Autodesk Inventor part; units mm, degrees
ref_plane "YZ Plane" through (0, 0, 0) normal (1, 0, 0) x (0, 1, 0)
ref_plane "XZ Plane" through (0, 0, 0) normal (0, 1, 0) x (-1, 0, 0)
ref_plane "XY Plane" through (0, 0, 0) normal (0, 0, 1) x (1, 0, 0)
sketch "スケッチ1" plane through (0, 0, 0) normal (0, 0, 1) x (1, 0, 0)
  line L0 (-28, -35) -> (28, -35) construction
  line L1 (28, -35) -> (28, 35) construction
  line L2 (28, 35) -> (-28, 35) construction
  line L3 (-28, 35) -> (-28, -35) construction
  line L4 (-28, -35) -> (28, 35) construction
  line L5 (28, -35) -> (-28, 35) construction
  line L6 (-28, 22.1) -> (-28, 35)
  line L7 (-28, 35) -> (28, 35)
  line L8 (28, 35) -> (28, 22.1)
  line L9 (-28, 20) -> (-33, 20)
  line L10 (-33, 20) -> (-33, -20)
  line L11 (-33, -20) -> (-28, -20)
  line L12 (-28, -22.1) -> (-28, -35)
  line L13 (-28, -35) -> (28, -35)
  line L14 (28, -35) -> (28, -22.1)
  line L15 (28, 20) -> (33, 20)
  line L16 (33, 20) -> (33, -20)
  line L17 (33, -20) -> (28, -20)
  arc A0 (-28, 20) -> (-28, 22.1) centre (-28, 21.05) ccw
  arc A1 (-28, -22.1) -> (-28, -20) centre (-28, -21.05) ccw
  arc A2 (28, -20) -> (28, -22.1) centre (28, -21.05) ccw
  line L18 (0, 0) -> (0, 35) construction
  line L19 (0, 0) -> (28, 0) construction
  arc A3 (28, 22.1) -> (28, 20) centre (28, 21.05) ccw
  dimension "d9" = 56
  dimension "d12" = 70
  dimension "d13" = 15
  dimension "d39" = 15
  dimension "d40" = 1.05
  dimension "d41" = 5
extrude "押し出し1" add sketch "スケッチ1" along normal blind 5
sketch "スケッチ2" plane through (0, 0, 5) normal (0, 0, 1) x (1, 0, 0)
  line L0 (-28, 35) -> (-28, 22.1)
  line L1 (28, 35) -> (-28, 35)
  line L2 (-67.7785, 43.014) -> (-28, 43.014)
  line L3 (-28, 43.014) -> (-28, -43.014)
  line L4 (-28, -43.014) -> (-67.7785, -43.014)
  line L5 (-67.7785, -43.014) -> (-67.7785, 43.014)
  line L6 (67.7785, 43.014) -> (28, 43.014)
  line L7 (28, 43.014) -> (28, -43.014)
  line L8 (28, -43.014) -> (67.7785, -43.014)
  line L9 (67.7785, -43.014) -> (67.7785, 43.014)
  line L10 (0, 0) -> (0, 35) construction
  line L11 (0, 0) -> (33, 0) construction
  line L12 (33, 20) -> (33, -20) construction
extrude "押し出し2" cut sketch "スケッチ2" against normal blind 2.5
sketch "スケッチ3" plane through (0, 0, 5) normal (0, 0, 1) x (1, 0, 0)
  line L0 (28, 35) -> (-28, 35)
  line L1 (-28, 35) -> (-28, 22.1)
  line L2 (-20, -27) -> (20, -27)
  line L3 (20, -27) -> (20, 27)
  line L4 (20, 27) -> (-20, 27)
  line L5 (-20, 27) -> (-20, -27)
  line L6 (-20, -27) -> (20, 27) construction
  line L7 (20, -27) -> (-20, 27) construction
  point P0 (0, 0)
  dimension "d47" = 8
  dimension "d48" = 8
extrude "押し出し3" cut sketch "スケッチ3" against normal blind 10
fillet "フィレット1" radius 10 4 edges at (-20, 27, 2.5) (20, 27, 2.5) (20, -27, 2.5) (-20, -27, 2.5)
equation "\"d12\" = d18"
equation "\"d13\" = d28"
equation "\"d39\" = d13"
equation "\"d47\" = d48"
properties part number "コックピット_2_サブフレーム_1" material "アセタール樹脂、黒"
Check sheet for the modelled part. Datum: model origin and axes. Units: mm. A direction names the side the tool comes from. Give positions to 0.01 mm unless a question says otherwise; leave off trailing zeros. Loops run counter-clockwise (first coordinate to the right, second up) from the corner with the lowest first, then second, coordinate; pieces in that order, holes last. Notation, with made-up numbers: M -27,78 L -23,78 A17 cw -23,90 Z; hole C -34.75,-22 d9. An arc over 180 degrees is marked long. Return JSON: item names as keys, results as strings. Group by question number.
1. Cross-section at D-D on y = 24.5. Record the boundary of the cut face in (x, z).
2. Mould release check, pull along X, two halves, no side actions. Record for faces 5 (the cylindrical face through (-26.95, 21.07, 2.46)), 6 (the flat face through (20, 0, 3)), 7 (the flat face through (30, 20, 1)): released by +X, released by -X, zero draft, split by the parting line, or undercut.
3. Tool access check on faces 1 (the flat face through (28, 29, 2)), 2 (the cylindrical face through (-16.99, -24.15, 2.46)), 3 (the flat face through (30, 0, 2.5)), 4 (the flat face through (28, -29, 2)). Record the directions out of +Z, -Z, +X, -X, +Y, -Y that give a thin tool (end or side, any length) a straight path to the whole face; none if there is none.
4. Cross-section at C-C on x = 16. Record the boundary of the cut face in (y, z), plus the area to 3 significant figures.
5. Cross-section at B-B on y = 14.5. Record the boundary of the cut face in (x, z).
6. Go/stop test with flat-tipped pins: pin 1 (2 mm diameter, centred on y = -0.5, z = 4, fed in from +X); pin 2 (12 mm diameter, centred on x = -13.5, y = -16.5, fed in from -Z); pin 3 (0.8 mm diameter, centred on y = 2, z = 3, fed in from -X); pin 4 (3 mm diameter, centred on x = -31, z = 1, fed in from +Y). Record where each tip stops, or that it passes through.
7. Thickness scan on L1, parallel to Y at x = 6, z = 2.4; L2, parallel to X at y = 9.5, z = 4.35; L3, parallel to X at y = -4, z = 1.5. Record the ranges inside material, lowest first.
8. Cross-section at A-A on z = 3.9. Record the boundary of the cut face in (x, y).
Return value:
{
 "1": {"outline": "M -28,0 L -16.61,0 L -16.61,5 L -28,5 Z; M 16.61,0 L 28,0 L 28,5 L 16.61,5 Z"},
 "2": {"face 5": "released by -X", "face 6": "undercut", "face 7": "zero draft"},
 "3": {"face 1": "+Z, -Z, +X, +Y", "face 2": "+Z, -Z", "face 3": "+Z, +X, +Y, -Y", "face 4": "+Z, -Z, +X, -Y"},
 "4": {"outline": "M -35,0 L -25,0 L -25,5 L -35,5 Z; M 25,0 L 35,0 L 35,5 L 25,5 Z", "area": "100 mm^2"},
 "5": {"outline": "M -33,0 L -20,0 L -20,5 L -28,5 L -28,2.5 L -33,2.5 Z; M 20,0 L 33,0 L 33,2.5 L 28,2.5 L 28,5 L 20,5 Z"},
 "6": {"pin 1": "x = 28", "pin 2": "through", "pin 3": "x = -28", "pin 4": "y = 20"},
 "7": {"L1": "-35 to -27, 27 to 35", "L2": "-28 to -20, 20 to 28", "L3": "-33 to -20, 20 to 33"},
 "8": {"outline": "M -28,-35 L 28,-35 L 28,-22.1 A1.05 cw 28,-20 L 28,20 A1.05 cw 28,22.1 L 28,35 L -28,35 L -28,22.1 A1.05 cw -28,20 L -28,-20 A1.05 cw -28,-22.1 Z; hole M -20,-17 A10 ccw -10,-27 L 10,-27 A10 ccw 20,-17 L 20,17 A10 ccw 10,27 L -10,27 A10 ccw -20,17 Z"}
}
